Read the model definition and answer for the solid it produces. Units are mm, in the model's axes. A direction names the side the tool comes from. Round coordinates to 2 decimals unless told otherwise and drop trailing zeros. Order: outer loops, then holes, each group sorted by start corner. A loop starts at its lowest first (then second) coordinate and runs counter-clockwise, first axis right, second up. Notation, with made-up numbers: (7, 55) -> (22, 55) arc R22 ccw to (22, 72) -> close; hole circle Ø11 at (68, -35). An arc over 180 degrees is marked (long way). One line per item, written item: value. Start each with the question number.
1. The mould has two halves that part along X. Classify faces 1 (the face through (-345, -229.963, -49)), 2 (the face through (-381.852, 209, -49)), 3 (the face through (-306.122, -208, -49)): released by +X, released by -X, zero draft, split by the parting line, or undercut.
2. Consider line 1 (Y direction, x = -343, z = 1203); line 2 (Z direction, x = -62, y = -140). Determine where each line is inside the solid, lowest interval first.
3. Section B-B (x = -25) is taken. Give the vertices of the cut face in (y, z).
4. For faces 4 (the face through (343, 229.963, -49)), 5 (the face through (-381.852, -208, -49)), 6 (the face through (-345, -186.803, -49)), 7 (the face through (381.852, 209, -49)), 8 (the face through (214, -247, 838)), determine the directions among +Z, -Z, +X, -X, +Y, -Y from which every point of the face is accessible in a straight line to the end or side of a thin tool.
5. Flat-ended cylindrical pins translate along their axes: pin 1 Ø22.5 at (x, z) = (328.5, -44.5) entering from -Y; pin 2 Ø4 at (x, y) = (-286.5, 147) entering from -Z; pin 3 Ø21.5 at (y, z) = (-218.5, -31.5) entering from +X. Find the tip coordinate at first contact, or state that the pin passes through.
6. Section A-A (y = -85) is taken. Give the vertices of the cut face in (x, z), then the cut area to 3 significant figures.
from build123d import *

# Parameters (mm, degrees)
F0_W     = 810
F0_H     = 500
F1_DEPTH = 1700
F2_W     = 75.7292719425
F2_H     = 43.1599973455
F3_DEPTH = 100
F4_W     = 317.8355082985
F4_H     = 1607.6748847961
F5_DEPTH = 3
F5_TAPER = -10


with BuildPart() as f1:
    # F0 (on Top) → F1 (new body)
    with BuildSketch(Plane.XY):
        Rectangle(F0_W, F0_H)
    extrude(amount=F1_DEPTH)

    # F2 (on face) → F3 (join)
    with BuildSketch(Plane(origin=(0, 0, 0), x_dir=(1, 0, 0), z_dir=(0, 0, -1))):
        with Locations((-343.9869582653, 208.3826959133)):
            Rectangle(F2_W, F2_H)
        with Locations((343.9869582653, 208.3826959133)):
            Rectangle(F2_W, F2_H)
        with Locations((343.9869582653, -208.3826959133)):
            Rectangle(F2_W, F2_H)
        with Locations((-343.9869582653, -208.3826959133)):
            Rectangle(F2_W, F2_H)
    extrude(amount=F3_DEPTH)

    # F4 (on face) → F5 (cut)
    with BuildSketch(Plane.XZ.offset(250)):
        with Locations((-211.9153991399, 850)):
            Rectangle(F4_W, F4_H)
        with Locations((211.9153991399, 850)):
            Rectangle(F4_W, F4_H)
    extrude(amount=-F5_DEPTH, taper=F5_TAPER, mode=Mode.SUBTRACT)


solid = f1.part
Answer:
1. face 1: zero draft
1. face 2: released by -X
1. face 3: undercut
2. line 1: -247 to 250
2. line 2: 0 to 1700
3. outline: (-250, 0) -> (250, 0) -> (250, 1700) -> (-250, 1700) -> close
4. face 4: -Z, +X, -X, +Y
4. face 5: -Z, -X, +Y, -Y
4. face 6: -Z, +X, -X
4. face 7: -Z, +X, +Y, -Y
4. face 8: -Y
5. pin 1: y = -229.96
5. pin 2: z = 0
5. pin 3: x = 381.85
6. outline: (-405, 0) -> (405, 0) -> (405, 1700) -> (-405, 1700) -> close
6. area: 1,380,000 mm^2
